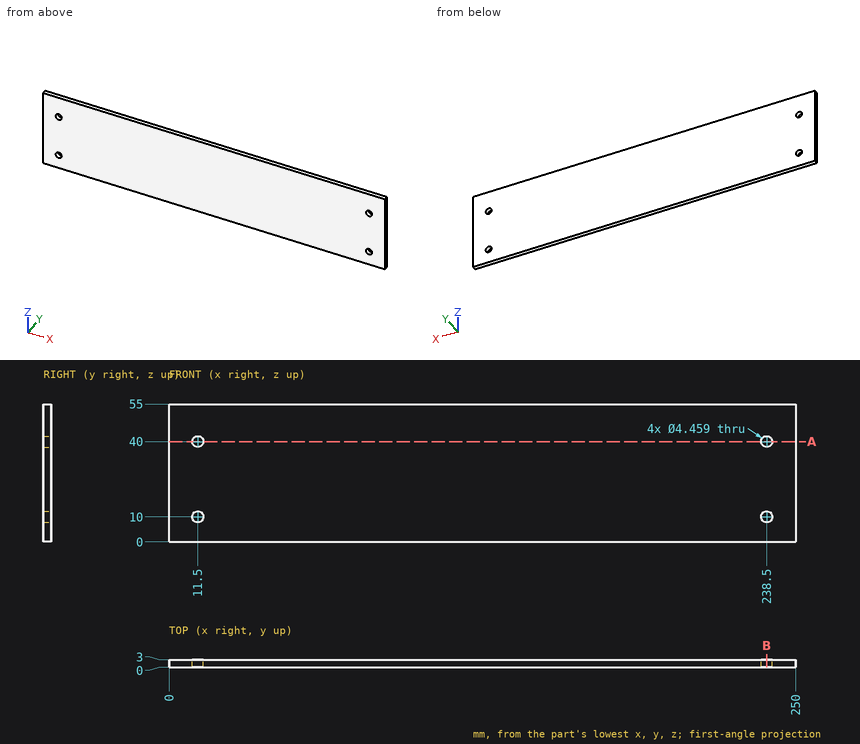
Answer from the drawing. Dimensions are ordinates in mm from the lowest x, y and z of the part. Give positions to 0.01 mm unless a question says otherwise; leave off trailing zeros. Write each loop counter-clockwise with the first axis right and the second up, starting at its lowest first coordinate (ties: lowest second). Pieces come first, ordered by that corner, then holes. Notation, with made-up numbers: (30, 89.5) - (43, 89.5) arc R12 ccw to (43, 93.5) - close; hole circle Ø3 at (40.5, 43). An arc over 180 degrees is marked (long way). Answer in a Markdown table with one row per item. Add a question column.
Item 1: Find the intervals of material crossed by L1, parallel to X at y = 2.2, z = 10; L2, parallel to Z at x = 238.5, y = 2.4, in increasing order.
Item 2: A flat-ended cylindrical pin translates along its axis: P1, Ø3.5, axis at x = 238.5, z = 10, coming from the +Y side. Find the tip coordinate at first contact, or state that the pin passes through.
Item 3: Section A-A, the plane z = 40 is taken. Write down the section's boundary in (x, y).
Item 4: Section B-B, the plane x = 238.5 is taken. Write down the section's boundary in (y, z), and give its area (3 significant figures).
Recorded:
| question | item | result |
|---|---|---|
| 1 | L1 | x = 0 to 9.27, 13.73 to 236.27, 240.73 to 250 |
| 1 | L2 | z = 0 to 7.77, 12.23 to 37.77, 42.23 to 55 |
| 2 | P1 | passes through |
| 3 | outline | (0, 0) - (9.27, 0) - (9.27, 3) - (0, 3) - close; (13.73, 0) - (236.27, 0) - (236.27, 3) - (13.73, 3) - close; (240.73, 0) - (250, 0) - (250, 3) - (240.73, 3) - close |
| 4 | outline | (0, 0) - (3, 0) - (3, 7.77) - (0, 7.77) - close; (0, 12.23) - (3, 12.23) - (3, 37.77) - (0, 37.77) - close; (0, 42.23) - (3, 42.23) - (3, 55) - (0, 55) - close |
| 4 | area | 138 mm2 |
